Input: part model. Units: mm. Frame: model coordinates. Face numbers are marked on the shaded views. A direction names the side the tool comes from. Coordinates: 2 decimals unless noted, no trailing zeros. Write each loop counter-clockwise with the first axis right and the second up, starting at its lowest first coordinate (ties: lowest second). Pieces come first, ordered by that corner, then holes. Notation, with made-up numbers: M 11.5,-33.5 L 33.5,-33.5 A17 ccw 33.5,-28.5 Z; hole C 68.25,-3 d3. An arc over 180 degrees is marked long. Write each question's results on one line, items separated by ' | '. Start each with the question number.
1. Pull-direction query (X, two-part tool) for the marked faces 1, 2 and 3; classes: +X half, -X half, draft (parallel to the pull), parting line (faces both ways), or undercut.
2. Section query C-C, the plane x = 130. Output: boundary loops of the cut face in (y, z), and give its area (3 significant figures).
3. Section query B-B, the plane y = 18. Output: boundary loops of the cut face in (x, z).
4. Set-up query: the marked faces 4, 5 and 6. Return all of +Z, -Z, +X, -X, +Y, -Y with unobstructed straight access to the full face (end or side cutting, diameter ignored); none if empty.
5. Section query D-D, the plane z = -22. Output: boundary loops of the cut face in (x, y), and give its area (3 significant figures).
6. First-contact query: pin 1 (3 mm diameter, centred on y = 34, z = -7, fed in from -X); pin 2 (8 mm diameter, centred on x = 48.5, z = -17, fed in from -Y); pin 3 (8 mm diameter, centred on x = 11, z = -15.5, fed in from +Y); pin 4 (5.5 mm diameter, centred on x = 130, z = -12, fed in from +Y). Flat tips, straight axial feed; report the tip coordinate or a pass-through.
7. Ray query, probe 1 along Z at (x, y) = (130, 22); probe 2 along X at (y, z) = (17, -7) (3 decimals); probe 3 along X at (y, z) = (13.5, -13.25). Return the intervals inside material, ascending.
8. Section query A-A, the plane y = 4.5. Output: boundary loops of the cut face in (x, z), and give its area (3 significant figures).
```python
from build123d import *

# Parameters (mm, degrees)
EXTRUDE_1_DEPTH          = 24
CUT_EXTRUDE_1_DEPTH      = 148.566933966
CUT_EXTRUDE_1_DEPTH_BACK = 20
SKETCH_2_R               = 4.5
CUT_EXTRUDE_2_DEPTH      = 10
CUT_EXTRUDE_2_DEPTH_BACK = 24
SKETCH_3_R               = 8


with BuildPart() as part:
    # 草图1 → 凸台-拉伸1 (new body)
    with BuildSketch(Plane.XY):
        with BuildLine():
            Line((0, 0), (0, 14))
            Line((0, 14), (15.83900126, 37.772379752))
            ThreePointArc((15.83900126, 37.772379752), (17.640116397, 39.408055056), (20, 40))
            Line((20, 40), (120, 40))
            ThreePointArc((120, 40), (122.359883603, 39.408055056), (124.16099874, 37.772379752))
            Line((124.16099874, 37.772379752), (140, 14))
            Line((140, 14), (140, 0))
            Line((140, 0), (120, 0))
            Line((120, 0), (120, 29))
            ThreePointArc((120, 29), (118.535533906, 32.535533906), (115, 34))
            Line((115, 34), (25, 34))
            ThreePointArc((25, 34), (21.464466094, 32.535533906), (20, 29))
            Line((20, 29), (20, 0))
            Line((20, 0), (0, 0))
        make_face()
    extrude(amount=-EXTRUDE_1_DEPTH)

    # 草图2 → 切除-拉伸1 (cut, two sides: drawn at the far end of the back side and taken through both)
    with BuildSketch(Plane.XZ.offset(-CUT_EXTRUDE_1_DEPTH_BACK)):
        with Locations(Location((10, -12, 0), (0, 0, 180))):
            Circle(SKETCH_2_R)
        with Locations(Location((130, -12, 0), (0, 0, 180))):
            Circle(SKETCH_2_R)
    extrude(amount=CUT_EXTRUDE_1_DEPTH + CUT_EXTRUDE_1_DEPTH_BACK, mode=Mode.SUBTRACT)

    # 草图3 → 切除-拉伸2 (cut, two sides: drawn at the far end of the back side and taken through both)
    with BuildSketch(Plane.XZ.offset(-20).offset(-CUT_EXTRUDE_2_DEPTH_BACK)):
        with Locations(Location((130, -12, 0), (0, 0, 223.124062677))):
            Circle(SKETCH_3_R)
        with Locations(Location((10, -12, 0), (0, 0, 316.875929093))):
            Circle(SKETCH_3_R)
    extrude(amount=CUT_EXTRUDE_2_DEPTH + CUT_EXTRUDE_2_DEPTH_BACK, mode=Mode.SUBTRACT)


solid = part.part
```
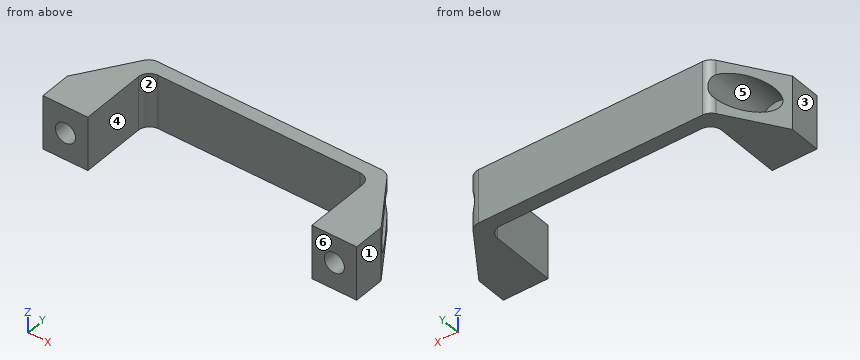
Answer:
1) face 1: +X half | face 2: undercut | face 3: -X half
2) outline: M 0,-24 L 29.01,-24 L 29.01,-20 L 10,-20 L 10,-16.5 L 0,-16.5 Z; M 0,-7.5 L 10,-7.5 L 10,-4 L 29.01,-4 L 29.01,0 L 0,0 Z | area: 302 mm^2
3) outline: M 2.67,-24 L 20,-24 L 20,0 L 2.67,0 L 2.67,-8.81 A8 cw long 2.67,-15.19 Z; M 120,-24 L 137.33,-24 L 137.33,-15.19 A8 cw long 137.33,-8.81 L 137.33,0 L 120,0 Z
4) face 4: +Z, -Z, -Y | face 5: +Y | face 6: +Z, -Z, +X, -X, -Y
5) outline: M 0,0 L 20,0 L 20,29 A5 cw 25,34 L 115,34 A5 cw 120,29 L 120,0 L 140,0 L 140,14 L 124.16,37.77 A5 ccw 120,40 L 20,40 A5 ccw 15.84,37.77 L 0,14 Z | area: 1,760 mm^2
6) pin 1: x = 14.66 | pin 2: y = 34 | pin 3: y = 10 | pin 4: through
7) probe 1: -24 to -20, -4 to 0 | probe 2: 1.999 to 3.755, 16.245 to 20, 120 to 123.755, 136.245 to 138.001 | probe 3: 0 to 2.1, 17.9 to 20, 120 to 122.1, 137.9 to 140
8) outline: M 0,-24 L 20,-24 L 20,0 L 0,0 Z; M 120,-24 L 140,-24 L 140,0 L 120,0 Z; hole C 10,-12 d9; hole C 130,-12 d9 | area: 833 mm^2
